from build123d import *

# Parameters (mm, degrees)
F1_DEPTH = 2.54
F2_R     = 1.905
F3_R     = 1.905
F3_R_2   = 1.27
F4_DEPTH = 2.541


with BuildPart() as f1:
    # F0 (on Front) → F1 (new body)
    with BuildSketch(Plane.XZ):
        with BuildLine():
            Line((0.335523, 3.795197), (0, 3.81))
            ThreePointArc((0, 3.81), (-0.084147, 3.809071), (-0.168252, 3.806283))
            ThreePointArc((-0.168252, 3.806283), (-3.806341, 0.166949), (-0.500857, -3.776936))
            Line((-0.500857, -3.776936), (0.168252, -3.806283))
            ThreePointArc((0.168252, -3.806283), (2.75292, -2.633919), (3.81, 0))
            ThreePointArc((3.81, 0), (2.8102, 2.572718), (0.335523, 3.795197))
        make_face()
        with BuildLine():
            ThreePointArc((0.335523, 3.795197), (0.167925, 3.806298), (0, 3.81))
            Line((0, 3.81), (0.335523, 3.795197))
        make_face()
        with BuildLine():
            ThreePointArc((-0.500857, -3.776936), (-3.806341, 0.166949), (-0.168252, 3.806283))
            Line((-0.168252, 3.806283), (-43.18, 1.905))
            Line((-43.18, 1.905), (-43.18, -1.905))
            Line((-43.18, -1.905), (-0.500857, -3.776936))
        make_face()
        with BuildLine():
            Line((43.18, 1.905), (0.335523, 3.795197))
            ThreePointArc((0.335523, 3.795197), (2.8102, 2.572718), (3.81, 0))
            ThreePointArc((3.81, 0), (2.75292, -2.633919), (0.168252, -3.806283))
            Line((0.168252, -3.806283), (43.18, -1.905))
            Line((43.18, -1.905), (43.18, 1.905))
        make_face()
        with BuildLine():
            Line((0.168252, -3.806283), (-0.500857, -3.776936))
            ThreePointArc((-0.500857, -3.776936), (-0.166949, -3.806341), (0.168252, -3.806283))
        make_face()
    extrude(amount=F1_DEPTH)

    # F2
    f2_edges = [f1.edges().sort_by_distance(p)[0] for p in [
        (43.18, -1.27, -1.905),
        (43.18, -1.27, 1.905),
        (-43.18, -1.27, 1.905),
        (-43.18, -1.27, -1.905),
    ]]
    fillet(f2_edges, radius=F2_R)

    # F3 (on face) → F4 (cut, through all)
    with BuildSketch(Plane.XZ.offset(2.54)):
        Circle(F3_R)
        with Locations((39.37, 0)):
            Circle(F3_R_2)
        with Locations((-41.275, -0.081723)):
            Circle(F3_R_2)
    extrude(amount=-F4_DEPTH, mode=Mode.SUBTRACT)


solid = f1.part
Model file for the job. Use its own axes, mm. Coordinates: 2 decimals unless noted, no trailing zeros. Loops run counter-clockwise (first coordinate to the right, second up) from the corner with the lowest first, then second, coordinate; pieces in that order, holes last. Notation, with made-up numbers: (35.5, -14.75) -> (70.5, -14.75) arc R10 ccw to (70.5, -6.75) -> close; hole circle Ø4 at (19, 70). An arc over 180 degrees is marked (long way). Use one line per item in the form item = value. Start each with the question number.
(1) Cut at B-B on x = 39.37. Give the cut face in (y, z), and give its area (3 significant figures).
(2) Cut at D-D on x = -21. Give the cut face in (y, z).
(3) Pull direction X, two halves, no side cores. Call faces 1 (the cylindrical face through (-0.41, -1.29, -1.86)), 2 (the flat face through (-1, 0, -2)), 3 (the flat face through (-21.22, -1.25, -2.87)), 4 (the cylindrical face through (-42.544, -1.288, -0.026)): pulls with the +X half, pulls with the -X half, needs draft (parallel to the pull), parting line crosses it, or undercut.
(4) Cut at C-C on z = -2.75. Give the cut face in (x, y), and give its area (3 significant figures).
(5) Probe probe 1 along X at (y, z) = (-0.9, 1); probe 2 along X at (y, z) = (-0.9, -0.75); probe 3 along Z at (x, y) = (39.37, -1). List the from-to ranges inside material, lowest first. Write a range as from..to.
(6) Cut at A-A on y = -1.6. Give the cut face in (x, z) (3 decimals), and give its area (3 significant figures).
(7) Flat gauge pin, fed straight in: pin 1 (1 mm diameter, centred on x = -2.5, y = -1, fed in from +Z). Where does the tip first touch, or does it go through?
Values:
q1.outline = (-2.54, -2.07) -> (0, -2.07) -> (0, -1.27) -> (-2.54, -1.27) -> close; (-2.54, 1.27) -> (0, 1.27) -> (0, 2.07) -> (-2.54, 2.07) -> close
q1.area = 4.08 mm2
q2.outline = (-2.54, -2.88) -> (0, -2.88) -> (0, 2.89) -> (-2.54, 2.89) -> close
q3.face_1 = undercut
q3.face_2 = needs draft
q3.face_3 = pulls with the -X half
q3.face_4 = undercut
q4.outline = (-23.91, -2.54) -> (24.06, -2.54) -> (24.06, 0) -> (-23.91, 0) -> close
q4.area = 122 mm2
q5.probe_1 = -42.94..-41.94, -40.61..-1.62, 1.62..38.59, 40.15..42.94
q5.probe_2 = -43.06..-42.35, -40.2..-1.75, 1.75..38.35, 40.39..43.06
q5.probe_3 = -2.07..-1.27, 1.27..2.07
q6.outline = (-43.18, -0.082) arc R1.905 ccw to (-41.358, -1.985) -> (-0.501, -3.777) arc R3.81 ccw to (0.168, -3.806) -> (41.359, -1.985) arc R1.905 ccw to (43.18, -0.082) -> (43.18, 0.082) arc R1.905 ccw to (41.359, 1.985) -> (0.336, 3.795) arc R3.809 ccw to (0, 3.81) arc R3.808 ccw to (-0.168, 3.806) -> (-41.359, 1.985) arc R1.905 ccw to (-43.18, 0.082) -> close; hole circle Ø2.54 at (-41.275, -0.082); hole circle Ø3.81 at (0, 0); hole circle Ø2.54 at (39.37, 0)
q6.area = 469 mm2
q7.pin_1 = 3.73
